The model under review builds one solid part; all positions refer to its coordinate system, in mm. Face numbers are marked on the shaded views. A direction names the side the tool comes from. Coordinates: 2 decimals unless noted, no trailing zeros. Order: outer loops, then holes, each group sorted by start corner. A loop starts at its lowest first (then second) coordinate and runs counter-clockwise, first axis right, second up.
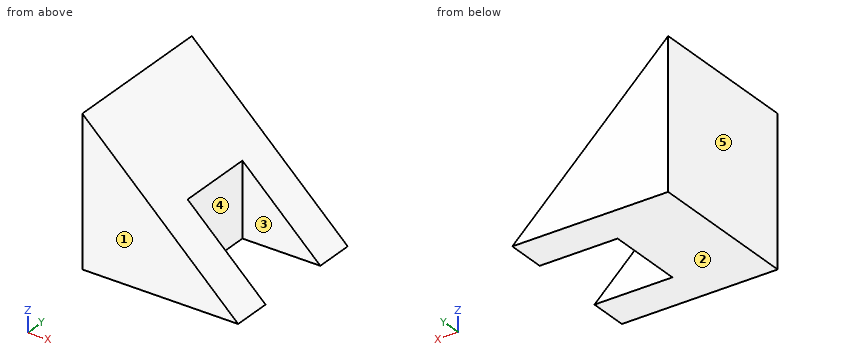
```python
from build123d import *

# Parameters (mm, degrees)
F1_DEPTH = 25.4
F3_START = -6.35
F3_DEPTH = 12.7


with BuildPart() as f1:
    # F0 (on Front) → F1 (new body)
    with BuildSketch(Plane.XZ):
        Polygon((0, 23.9633341665), (0, 0), (25.4, 0), align=None)
    extrude(amount=F1_DEPTH)

    # F2 (on face) → F3 (cut)
    with BuildSketch(Plane.XZ.offset(25.4).offset(F3_START)):
        Polygon((25.4, 0), (12.7, 11.9816670832), (12.7, 0), align=None)
    extrude(amount=-F3_DEPTH, mode=Mode.SUBTRACT)


solid = f1.part
```
(1) We need section C-C, the plane x = 19.5. Write out the cut boundary in (y, z).
A:
outline: (-25.4, 0) - (-19.05, 0) - (-19.05, 5.57) - (-25.4, 5.57) - close; (-6.35, 0) - (0, 0) - (0, 5.57) - (-6.35, 5.57) - close
(2) We need section A-A, the plane x = 14.25. Write out the cut boundary in (y, z).
A:
outline: (-25.4, 0) - (-19.05, 0) - (-19.05, 10.52) - (-25.4, 10.52) - close; (-6.35, 0) - (0, 0) - (0, 10.52) - (-6.35, 10.52) - close
(3) Machinability: for the marked faces 4 and 5, which of the approach directions +Z, -Z, +X, -X, +Y, -Y give a long, thin tool a straight path to every point of the face, cutting with its end or side? Answer none if there is none.
A:
face 4: +Z, -Z, +X
face 5: +Z, -Z, -X, +Y, -Y
(4) We need section D-D, the plane y = -13. Write out the cut boundary in (x, z).
A:
outline: (0, 0) - (12.7, 0) - (12.7, 11.98) - (0, 23.96) - close
(5) Wall thickness on probe 1 along Y at (x, z) = (17.5, 6); probe 2 along X at (y, z) = (-13.25, 10.25); probe 3 along Z at (x, y) = (14.25, -23.75): over which ranges is each line inside the solid? List them lowest first.
A:
probe 1: y = -25.4 to -19.05, -6.35 to 0
probe 2: x = 0 to 12.7
probe 3: z = 0 to 10.52
(6) For pin 1 Ø6 at (x, z) = (18.5, 6.5) entering from +Y; pin 2 Ø3.5 at (x, z) = (21.5, 6.5) entering from -Y; pin 3 Ø6 at (y, z) = (-20.5, 6) entering from +X; pin 4 Ø9.5 at (y, z) = (-10, 5) entering from +X, all flat-tipped, find the tip position at first contact; note any pin that passes through.
A:
pin 1: stops at y = 0
pin 2: passes through
pin 3: stops at x = 22.22
pin 4: stops at x = 23.32
(7) Draft analysis for pull direction Y (two halves, no side actions). For the marked faces 1, 2 and 3, state which applies: released by +Y, released by -Y, zero draft, split by the parting line, or undercut.
A:
face 1: released by -Y
face 2: zero draft
face 3: undercut
(8) We need section B-B, the plane z = 10.75. Write out the cut boundary in (x, y), and give its area (3 significant figures).
A:
outline: (0, -25.4) - (14.01, -25.4) - (14.01, -19.05) - (12.7, -19.05) - (12.7, -6.35) - (14.01, -6.35) - (14.01, 0) - (0, 0) - close
area: 339 mm2
